Build history of the part. All positions in model axes, mm. A direction names the side the tool comes from. Round coordinates to 2 decimals unless told otherwise and drop trailing zeros. Loops run counter-clockwise (first coordinate to the right, second up) from the corner with the lowest first, then second, coordinate; pieces in that order, holes last. Notation, with made-up numbers: (50.5, 30) - (67.5, 30) arc R20 cw to (67.5, 46) - close; hole circle Ø6 at (47.5, -38.5). An arc over 180 degrees is marked (long way). Put each result on its own line as item: value. Start each with the question number.
Autodesk Inventor part; units mm, degrees
ref_plane "YZ Plane" through (0, 0, 0) normal (1, 0, 0) x (0, 1, 0)
ref_plane "XZ Plane" through (0, 0, 0) normal (0, 1, 0) x (-1, 0, 0)
ref_plane "XY Plane" through (0, 0, 0) normal (0, 0, 1) x (1, 0, 0)
sketch "Sketch1" plane through (0, 0, 0) normal (0, 0, 1) x (1, 0, 0)
  line L0 (0, -8.9) -> (0, 0)
  line L1 (0, 0) -> (20.15, 0)
  line L2 (20.15, 0) -> (20.15, -6.4)
  line L3 (20.15, -6.4) -> (12.2, -6.4)
  line L4 (12.2, -6.4) -> (12.2, -7.4)
  line L5 (12.2, -7.4) -> (7, -7.4)
  line L6 (7, -7.4) -> (7, -8.9)
  line L7 (7, -8.9) -> (6.45, -8.9)
  line L8 (6.45, -8.9) -> (6.45, -12.85)
  line L9 (6.45, -12.85) -> (5.45, -12.85)
  line L10 (5.45, -12.85) -> (5.45, -8.9)
  line L11 (5.45, -8.9) -> (1.55, -8.9)
  line L12 (1.55, -8.9) -> (1.55, -12.85)
  line L13 (1.55, -12.85) -> (0.55, -12.85)
  line L14 (0.55, -12.85) -> (0.55, -8.9)
  line L15 (0.55, -8.9) -> (0, -8.9)
  dimension "d0" = 20.15
  dimension "d1" = 1
  dimension "d2" = 7
  dimension "d3" = 3.9
  dimension "d4" = 1.5
  dimension "d5" = 1
  dimension "d6" = 7.4
  dimension "d7" = 12.2
  dimension "d9" = 12.85
extrude "Extrusion1" add sketch "Sketch1" along normal blind 0.87
sketch "Sketch2" plane through (0, 0, 0.87) normal (0, 0, 1) x (1, 0, 0)
  line L0 (0, 0) -> (20.15, 0)
  line L1 (20.15, -6.4) -> (12.2, -6.4)
  line L2 (20.15, 0) -> (20.15, -6.4)
  line L3 (15.75, -3.2) -> (15.75, 0) construction
  line L4 (15.75, -3.2) -> (15.75, -6.4) construction
  dimension "d13" = 4.4
hole "Hole1" at (15.75, -3.2, 0.87) direction (0, 0, -1) diameter 1.85 end through all
chamfer "Chamfer1" distance 0.5 angle 45 2 edges at (20.15, -6.4, 0.435) (20.15, 0, 0.435)
chamfer "Chamfer2" distance 0.2 angle 45 2 edges at (20.15, -3.2, 0.87) (20.15, -3.2, 0)
chamfer "Chamfer3" distance 1 angle 45 1 edges at (0, 0, 0.435)
properties part number "Spike Male Terminal" material "Steel, Mild"
Item 1: Slice it at A-A (y = -11). Give the cut face in (x, z).
Item 2: Slice it at B-B (x = 15.75). Give the cut face in (y, z) (3 decimals), plus the area to 3 significant figures.
Item 3: Which spindle directions (+Z, -Z, +X, -X, +Y, -Y) get a long thin tool onto all of the face, cutting with end or side? Do faces 1 (the flat face through (0.55, -10.9, 0.4)), 2 (the flat face through (1.1, -12.85, 0.4)), 3 (the flat face through (6.45, -10.8, 0.4)), 4 (the flat face through (0, -5, 0.4)), 5 (the flat face through (1.55, -10.8, 0.4)). Say none if no direction does.
Item 4: Slice it at C-C (z = 0.35). Give the cut face in (x, y) (3 decimals).
Item 5: Slice it at D-D (y = -3.2). Give the cut face in (x, z) (3 decimals), plus the area to 3 significant figures.
Item 6: Drill centre lines: probe 1 along Y at (x, z) = (15.75, 0.5) (3 decimals); probe 2 along X at (y, z) = (-11.5, 0.5); probe 3 along Y at (x, z) = (3.5, 0.15). Where is each one in solid material? Low to high. Write a range as [from, to].
Item 7: Two-plate mould, pull along Y, no slides. Class faces 6 (the cylindrical face through (14.833, -3.08, 0.429)), 7 (the flat face through (10.2, 0, 0.4)), 8 (the flat face through (7, -8.1, 0.4)): pulls with the +Y half, pulls with the -Y half, needs draft (parallel to the pull), parting line crosses it, or undercut.
Computed values:
1. outline: (0.55, 0) - (1.55, 0) - (1.55, 0.87) - (0.55, 0.87) - close; (5.45, 0) - (6.45, 0) - (6.45, 0.87) - (5.45, 0.87) - close
2. outline: (-6.4, 0) - (-4.125, 0) - (-4.125, 0.87) - (-6.4, 0.87) - close; (-2.275, 0) - (0, 0) - (0, 0.87) - (-2.275, 0.87) - close
2. area: 3.96 mm^2
3. face 1: +Z, -Z, -X, -Y
3. face 2: +Z, -Z, +X, -X, -Y
3. face 3: +Z, -Z, +X, -Y
3. face 4: +Z, -Z, -X, +Y, -Y
3. face 5: +Z, -Z, -Y
4. outline: (0, -8.9) - (0.55, -8.9) - (0.55, -12.85) - (1.55, -12.85) - (1.55, -8.9) - (5.45, -8.9) - (5.45, -12.85) - (6.45, -12.85) - (6.45, -8.9) - (7, -8.9) - (7, -7.4) - (12.2, -7.4) - (12.2, -6.4) - (19.65, -6.4) - (20.15, -5.9) - (20.15, -0.5) - (19.65, 0) - (1, 0) - (0, -1) - close; hole circle Ø1.85 at (15.75, -3.2)
5. outline: (0, 0) - (14.825, 0) - (14.825, 0.87) - (0, 0.87) - close; (16.675, 0) - (19.95, 0) - (20.15, 0.2) - (20.15, 0.67) - (19.95, 0.87) - (16.675, 0.87) - close
5. area: 15.9 mm^2
6. probe 1: y = [-6.4, -4.125], [-2.275, 0]
6. probe 2: x = [0.55, 1.55], [5.45, 6.45]
6. probe 3: y = [-8.9, 0]
7. face 6: undercut
7. face 7: pulls with the +Y half
7. face 8: needs draft
